```python
from build123d import *

# Parameters (mm, degrees)
SCHIZZO1_W                   = 52
SCHIZZO1_H                   = 25.4
ESTRUSIONE_ESTRUSIONE1_DEPTH = 9
FORO_PER_VITE_M2_1_D         = 2.4
SCHIZZO5_R                   = 5
ESTRUSIONE_ESTRUSIONE2_DEPTH = 1
SCHIZZO6_W                   = 8
SCHIZZO6_H                   = 0.5
ESTRUSIONE_ESTRUSIONE3_DEPTH = 0.5
SCHIZZO7_R                   = 1.375
ESTRUSIONE_ESTRUSIONE4_DEPTH = 1
CUPOLA1_FACE_RADIUS          = 1.375
CUPOLA1_HEIGHT               = 1.375
CUPOLA2_FACE_RADIUS          = 1.375
CUPOLA2_HEIGHT               = 1.375
CUPOLA3_FACE_RADIUS          = 1.375
CUPOLA3_HEIGHT               = 1.375


with BuildPart() as part:
    # Schizzo1 → Estrusione-Estrusione1 (new body)
    with BuildSketch(Plane.XY):
        Rectangle(SCHIZZO1_W, SCHIZZO1_H)
    extrude(amount=ESTRUSIONE_ESTRUSIONE1_DEPTH)

    # Foro per Vite M2-1 (through all)
    with Locations(Plane.XY.offset(9)):
        with Locations((-23.725, 10.44), (-23.725, -10.44), (23.725, -10.44), (23.725, 10.44)):
            Hole(FORO_PER_VITE_M2_1_D / 2)

    # Schizzo5 → Estrusione-Estrusione2 (add)
    with BuildSketch(Plane.XY.offset(9)):
        with Locations(Location((-15, 0, 0), (0, 0, 180))):
            Circle(SCHIZZO5_R)
        with Locations(Location((15, 0, 0), (0, 0, 180))):
            Circle(SCHIZZO5_R)
    extrude(amount=ESTRUSIONE_ESTRUSIONE2_DEPTH)

    # Schizzo6 → Estrusione-Estrusione3 (add)
    with BuildSketch(Plane.XY.offset(9)):
        with Locations((9, 11.7)):
            Rectangle(SCHIZZO6_W, SCHIZZO6_H)
    extrude(amount=ESTRUSIONE_ESTRUSIONE3_DEPTH)

    # Schizzo7 → Estrusione-Estrusione4 (add)
    with BuildSketch(Plane.XY.offset(9)):
        with Locations(Location((-23.5, 0, 0), (0, 0, 180))):
            Circle(SCHIZZO7_R)
        with Locations(Location((23.5, 0, 0), (0, 0, 180))):
            Circle(SCHIZZO7_R)
        with Locations(Location((0, 0, 0), (0, 0, 180))):
            Circle(SCHIZZO7_R)
    extrude(amount=ESTRUSIONE_ESTRUSIONE4_DEPTH)

    # Cupola1: a dome of height H over a round flat face of radius A is a cap of a sphere of radius (A * A + H * H) / (2 * H)
    cupola1_r = (CUPOLA1_FACE_RADIUS * CUPOLA1_FACE_RADIUS + CUPOLA1_HEIGHT * CUPOLA1_HEIGHT) / (2 * CUPOLA1_HEIGHT)
    cupola1_base = Plane((-23.5, 0, 10), z_dir=(0, 0, 1))
    with Locations(cupola1_base.offset(CUPOLA1_HEIGHT - cupola1_r)):
        cupola1_ball = Sphere(cupola1_r, mode=Mode.PRIVATE)
    add(split(cupola1_ball, bisect_by=cupola1_base, keep=Keep.TOP, mode=Mode.PRIVATE))

    # Cupola2: a dome of height H over a round flat face of radius A is a cap of a sphere of radius (A * A + H * H) / (2 * H)
    cupola2_r = (CUPOLA2_FACE_RADIUS * CUPOLA2_FACE_RADIUS + CUPOLA2_HEIGHT * CUPOLA2_HEIGHT) / (2 * CUPOLA2_HEIGHT)
    cupola2_base = Plane((0, 0, 10), z_dir=(0, 0, 1))
    with Locations(cupola2_base.offset(CUPOLA2_HEIGHT - cupola2_r)):
        cupola2_ball = Sphere(cupola2_r, mode=Mode.PRIVATE)
    add(split(cupola2_ball, bisect_by=cupola2_base, keep=Keep.TOP, mode=Mode.PRIVATE))

    # Cupola3: a dome of height H over a round flat face of radius A is a cap of a sphere of radius (A * A + H * H) / (2 * H)
    cupola3_r = (CUPOLA3_FACE_RADIUS * CUPOLA3_FACE_RADIUS + CUPOLA3_HEIGHT * CUPOLA3_HEIGHT) / (2 * CUPOLA3_HEIGHT)
    cupola3_base = Plane((23.5, 0, 10), z_dir=(0, 0, 1))
    with Locations(cupola3_base.offset(CUPOLA3_HEIGHT - cupola3_r)):
        cupola3_ball = Sphere(cupola3_r, mode=Mode.PRIVATE)
    add(split(cupola3_ball, bisect_by=cupola3_base, keep=Keep.TOP, mode=Mode.PRIVATE))


solid = part.part
```
The model under review builds one solid part; all positions refer to its coordinate system, in mm. A direction names the side the tool comes from. Round coordinates to 2 decimals unless told otherwise and drop trailing zeros. Loops run counter-clockwise (first coordinate to the right, second up) from the corner with the lowest first, then second, coordinate; pieces in that order, holes last. Notation, with made-up numbers: (3, 8) -> (41, 8) arc R12 cw to (41, 16) -> close; hole circle Ø7 at (74.25, -12). An arc over 180 degrees is marked (long way). Answer as a JSON object with one key per item and string values. Group by question number.
1) For line 1 (X direction, y = -9.75, z = 8.5); line 2 (Z direction, x = 7, y = -11); line 3 (Z direction, x = -15, y = -0.75), list the stretches that pass through material, from the lowest coordinate up. Write a range as [from, to].
2) We need section B-B on x = 11. Write out the cut boundary in (y, z).
3) We need section A-A on y = 10.44. Write out the cut boundary in (x, z) (3 decimals), then the cut area to 3 significant figures.
4) We need section D-D on y = 3. Write out the cut boundary in (x, z), then the cut area to 3 significant figures.
5) Mouldability with a two-part tool opening along Y and no side actions: class faces 4 (the face through (-24.87, -10.08, 4.44)), 5 (the face through (-22.126, -0.06, 9.493)), 6 (the face through (0, 0, 0)) as released by +Y, released by -Y, zero draft, split by the parting line, or undercut.
6) For faces 1 (the face through (0.3, 1.34, 9.49)), 2 (the face through (22.58, -10.08, 4.44)), 3 (the face through (15, 0, 10)), list the 3-axis set-ups (+Z, -Z, +X, -X, +Y, -Y) from which the entire face can be reached by the end or side of a thin tool; tool diameter is ignored.
7) We need section C-C on x = -23.5. Write out the cut boundary in (y, z) (3 decimals), then the cut area to 3 significant figures.
8) For pin 1 Ø3 at (x, y) = (-23.725, -10.44) entering from +Z; pin 2 Ø1 at (x, y) = (-1.5, -0.5) entering from +Z; pin 3 Ø5 at (x, y) = (17.5, -2) entering from +Z, all flat-tipped, find the tip position at first contact; note any pin that passes through.
Result set:
{
 "1": {"line 1": "[-26, -24.71], [-22.74, 22.74], [24.71, 26]", "line 2": "[0, 9]", "line 3": "[0, 10]"},
 "2": {"outline": "(-12.7, 0) -> (12.7, 0) -> (12.7, 9) -> (11.95, 9) -> (11.95, 9.5) -> (11.45, 9.5) -> (11.45, 9) -> (3, 9) -> (3, 10) -> (-3, 10) -> (-3, 9) -> (-12.7, 9) -> close"},
 "3": {"outline": "(-26, 0) -> (-24.925, 0) -> (-24.925, 9) -> (-26, 9) -> close; (-22.525, 0) -> (22.525, 0) -> (22.525, 9) -> (-22.525, 9) -> close; (24.925, 0) -> (26, 0) -> (26, 9) -> (24.925, 9) -> close", "area": "425 mm²"},
 "4": {"outline": "(-26, 0) -> (26, 0) -> (26, 9) -> (19, 9) -> (19, 10) -> (11, 10) -> (11, 9) -> (-11, 9) -> (-11, 10) -> (-19, 10) -> (-19, 9) -> (-26, 9) -> close", "area": "484 mm²"},
 "5": {"face 4": "undercut", "face 5": "split by the parting line", "face 6": "zero draft"},
 "6": {"face 1": "+Z", "face 2": "+Z, -Z", "face 3": "+Z, +Y, -Y"},
 "7": {"outline": "(-12.7, 0) -> (-11.619, 0) -> (-11.619, 9) -> (-12.7, 9) -> close; (-9.261, 0) -> (9.261, 0) -> (9.261, 9) -> (1.375, 9) -> (1.375, 10) arc R1.375 ccw to (-1.375, 10) -> (-1.375, 9) -> (-9.261, 9) -> close; (11.619, 0) -> (12.7, 0) -> (12.7, 9) -> (11.619, 9) -> close", "area": "192 mm²"},
 "8": {"pin 1": "z = 9", "pin 2": "z = 10.85", "pin 3": "z = 10"}
}
